Job drawing, mm, ordinate dimensions from the low corner. One solid piece. A direction names the side the tool comes from. Coordinates: 2 decimals unless noted, no trailing zeros. Order: outer loops, then holes, each group sorted by start corner. A loop starts at its lowest first (then second) coordinate and runs counter-clockwise, first axis right, second up. Notation, with made-up numbers: (42.5, 67.25) - (89.5, 67.25) arc R23 ccw to (89.5, 83.25) - close; hole circle Ø7 at (-11.75, 85). An arc over 180 degrees is marked (long way). Use one line per item in the form item = value.
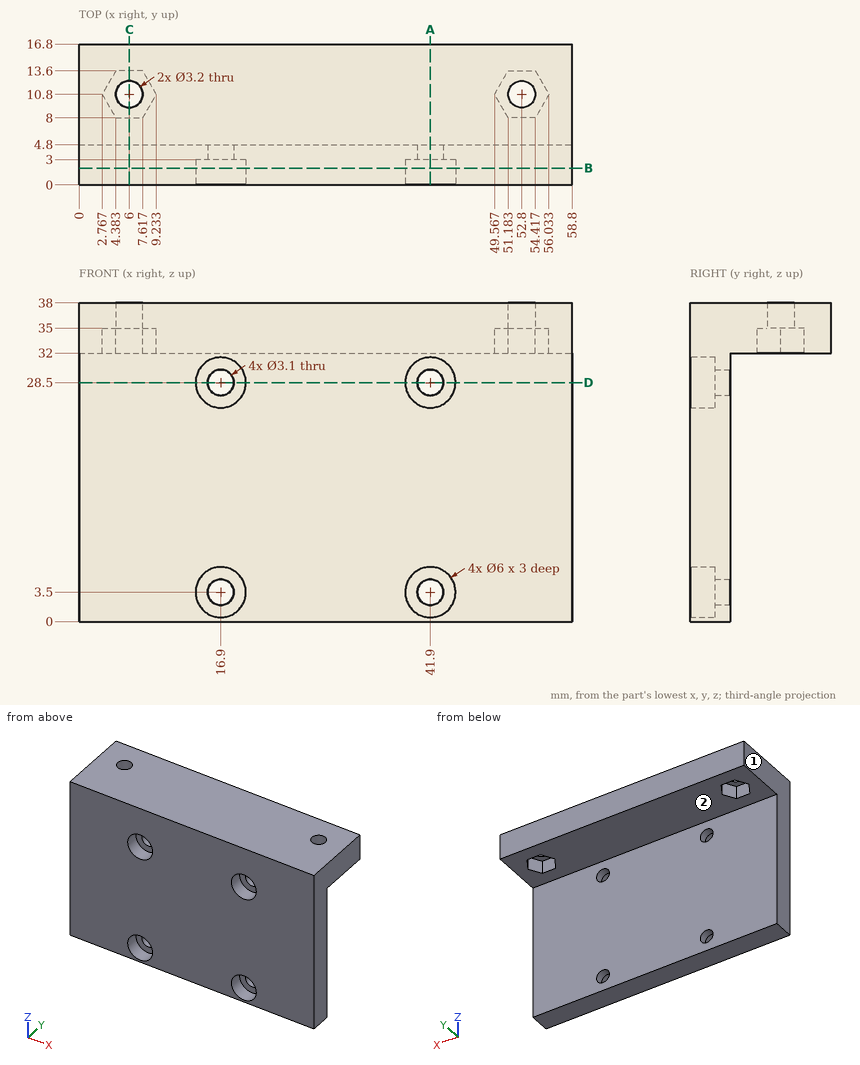
Item 1: Cut at C-C, the plane x = 6. Write the cut outline in (y, z), plus the area to 3 significant figures.
Derived:
outline = (0, 0) - (4.8, 0) - (4.8, 32) - (8, 32) - (8, 35) - (9.2, 35) - (9.2, 38) - (0, 38) - close; (12.4, 35) - (13.6, 35) - (13.6, 32) - (16.8, 32) - (16.8, 38) - (12.4, 38) - close
area = 228 mm²
Item 2: Drop flat-ended pins along their axis: pin 1 (7 mm diameter, centred on x = 41.9, z = 3.5, fed in from +Y); pin 2 (6 mm diameter, centred on x = 5, y = 11, fed in from -Z); pin 3 (6.5 mm diameter, centred on x = 15.5, z = 28, fed in from -Y); pin 4 (4 mm diameter, centred on x = 52.8, y = 10.8, fed in from -Z). Give the stop position or say it passes through.
Derived:
pin_1 = 4.8
pin_2 = 32
pin_3 = 0
pin_4 = 35
Item 3: Cut at D-D, the plane z = 28.5. Write the cut outline in (x, y).
Derived:
outline = (0, 0) - (13.9, 0) - (13.9, 3) - (15.35, 3) - (15.35, 4.8) - (0, 4.8) - close; (18.45, 3) - (19.9, 3) - (19.9, 0) - (38.9, 0) - (38.9, 3) - (40.35, 3) - (40.35, 4.8) - (18.45, 4.8) - close; (43.45, 3) - (44.9, 3) - (44.9, 0) - (58.8, 0) - (58.8, 4.8) - (43.45, 4.8) - close
Item 4: Drill centre lines: line 1 (X direction, y = 3.4, z = 3.5); line 2 (X direction, y = 2.3, z = 3.5); line 3 (Z direction, x = 30.5, y = 12.25). Where is each one in solid material? Low to high. Write a range as [from, to].
Derived:
line_1 = [0, 15.35], [18.45, 40.35], [43.45, 58.8]
line_2 = [0, 13.9], [19.9, 38.9], [44.9, 58.8]
line_3 = [32, 38]
Item 5: Cut at B-B, the plane y = 2. Write the cut outline in (x, z), plus the area to 3 significant figures.
Derived:
outline = (0, 0) - (58.8, 0) - (58.8, 38) - (0, 38) - close; hole circle Ø6 at (16.9, 3.5); hole circle Ø6 at (16.9, 28.5); hole circle Ø6 at (41.9, 3.5); hole circle Ø6 at (41.9, 28.5)
area = 2,120 mm²
Item 6: Cut at A-A, the plane x = 41.9. Write the cut outline in (y, z), plus the area to 3 significant figures.
Derived:
outline = (0, 0) - (4.8, 0) - (4.8, 1.95) - (3, 1.95) - (3, 0.5) - (0, 0.5) - close; (0, 6.5) - (3, 6.5) - (3, 5.05) - (4.8, 5.05) - (4.8, 26.95) - (3, 26.95) - (3, 25.5) - (0, 25.5) - close; (0, 31.5) - (3, 31.5) - (3, 30.05) - (4.8, 30.05) - (4.8, 32) - (16.8, 32) - (16.8, 38) - (0, 38) - close
area = 207 mm²
Item 7: 3-axis set-ups, long thin cutter, end or side, ignore diameter. For the marked faces 1 and 2: which of +Z, -Z, +X, -X, +Y, -Y reach the whole face in a straight line?
Derived:
face_1 = +Z, -Z, -X, +Y, -Y
face_2 = -Z, +X, -X, +Y
